Geometry check sheet. Reference: the model listing, model coordinates, mm. Face numbers are marked on the shaded views. Coordinates: 2 decimals unless noted, no trailing zeros. Order: outer loops, then holes, each group sorted by start corner. A loop starts at its lowest first (then second) coordinate and runs counter-clockwise, first axis right, second up. Notation, with made-up numbers: (-3, 80.25) - (4, 80.25) arc R22 ccw to (4, 117.25) - close; hole circle Ø11 at (-9, -39.5). An arc over 180 degrees is marked (long way). Put each result on its own line as item: value.
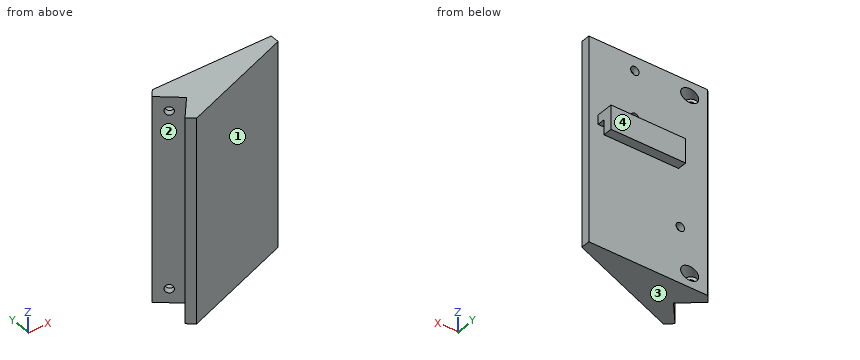
from build123d import *

# Parameters (mm, degrees)
EXTRUDE_1_DEPTH     = 65
EXTRUDE_2_DEPTH     = 5
EXTRUDE_4_DEPTH     = 8
SKETCH_9_R          = 2.3
CUT_EXTRUDE_4_DEPTH = 3.5
CUT_EXTRUDE_6_DEPTH = 14
EXTRUDE_5_DEPTH     = 40
HOLE_WIZARD_M4_1_D  = 4.5
CUT_EXTRUDE_START   = -3.5
SKETCH_17_R         = 3.75
CUT_EXTRUDE_7_DEPTH = 51.05954578
F_4_0MM_1_D         = 4.6
F_4_0MM_1_DEPTH     = 3.5
CUT_EXTRUDE_8_DEPTH = 5


with BuildPart() as part:
    # ｽｹｯﾁ1 → ﾎﾞｽ - 押し出し1 (new body)
    with BuildSketch(Plane.XY):
        Polygon((0, 0), (9.641814145, 11.490666647), (-1.848852501, 21.132480792), (1.365085547, 24.962703008), (65.946194887, 24.962703008), (65.946194887, 19.962703008), (3.830222216, -3.213938048), align=None)
    extrude(amount=EXTRUDE_1_DEPTH)

    # ｽｹｯﾁ6 → ﾎﾞｽ - 押し出し2 (add)
    with BuildSketch(Plane.XY.offset(65)):
        Polygon((0, 0), (3.830222216, -3.213938048), (65.946194887, 19.962703008), (65.946194887, 34.162703008), (9.084802154, 34.162703008), (-1.848852501, 21.132480792), (9.641814145, 11.490666647), align=None)
    extrude(amount=EXTRUDE_2_DEPTH)

    # ｽｹｯﾁ8 → ﾎﾞｽ - 押し出し4 (add)
    with BuildSketch(Plane(origin=(0, 0, 65), x_dir=(-1, 0, 0), z_dir=(0, 0, -1))):
        Polygon((-65.946194887, 34.162703008), (-65.946194887, 29.162703008), (-4.889303998, 29.162703008), (-9.084802154, 34.162703008), align=None)
    extrude(amount=EXTRUDE_4_DEPTH)

    # ｽｹｯﾁ9 → ｶｯﾄ - 押し出し4 (cut)
    with BuildSketch(Plane(origin=(0, 24.962703008, 0), x_dir=(1, 0, 0), z_dir=(0, 1, 0))):
        with Locations((16.255085547, -30)):
            Circle(SKETCH_9_R)
    extrude(amount=-CUT_EXTRUDE_4_DEPTH, mode=Mode.SUBTRACT)

    # ｽｹｯﾁ11 → ｶｯﾄ - 押し出し6 (cut, through all)
    with BuildSketch(Plane(origin=(0, 0, 57), x_dir=(-1, 0, 0), z_dir=(0, 0, -1))):
        Polygon((-1.365085547, 24.962703008), (-9.084802154, 34.162703008), (-20.364802154, 34.162703008), (-20.364802154, 24.962703008), align=None)
    extrude(amount=-CUT_EXTRUDE_6_DEPTH, mode=Mode.SUBTRACT)

    # ｽｹｯﾁ12 → ﾎﾞｽ - 押し出し5 (add)
    with BuildSketch(Plane.XY.offset(70)):
        Polygon((0, 0), (3.830222216, -3.213938048), (65.946194887, 19.962703008), (65.946194887, 24.962703008), (1.365085547, 24.962703008), (-1.848852501, 21.132480792), (9.641814145, 11.490666647), align=None)
    extrude(amount=EXTRUDE_5_DEPTH)

    # M4 すきま穴1 (through all)
    with Locations(Plane(origin=(9.641814145, 11.490666647, 0), x_dir=(-0.766044443, 0.64278761, 0), z_dir=(-0.64278761, -0.766044443, 0))):
        with Locations((7.5, -102.5), (7.5, -7.5)):
            Hole(HOLE_WIZARD_M4_1_D / 2)

    # ｽｹｯﾁ17 → ｶｯﾄ - 押し出し7 (cut, through all)
    with BuildSketch(Plane(origin=(9.641814145, 11.490666647, 0), x_dir=(0.766044443, -0.64278761, 0), z_dir=(-0.64278761, -0.766044443, 0)).offset(CUT_EXTRUDE_START)):
        with Locations((-7.5, 102.5)):
            Circle(SKETCH_17_R)
        with Locations((-7.5, 7.5)):
            Circle(SKETCH_17_R)
    extrude(amount=-CUT_EXTRUDE_7_DEPTH, mode=Mode.SUBTRACT)

    # Ø4.0mm ﾀﾞｳｴﾙ穴1
    with Locations(Plane(origin=(0, 24.962703008, 0), x_dir=(1, 0, 0), z_dir=(0, 1, 0))):
        with Locations((40.946194887, -77.5), (40.946194887, -102.5)):
            Hole(F_4_0MM_1_D / 2, depth=F_4_0MM_1_DEPTH)

    # ｽｹｯﾁ20 → ｶｯﾄ - 押し出し8 (cut)
    with BuildSketch(Plane(origin=(65.946194887, 0, 0), x_dir=(0, 0, -1), z_dir=(1, 0, 0))):
        Polygon((-70, 24.962703008), (-65, 24.962703008), (-65, 29.162703008), (-57, 29.162703008), (-57, 34.162703008), (-70, 34.162703008), align=None)
    extrude(amount=-CUT_EXTRUDE_8_DEPTH, mode=Mode.SUBTRACT)


solid = part.part
Q1. Section check C-C on x = 25. Record the boundary of the cut face in (y, z), then the cut area to 3 significant figures.
Answer block:
outline: (4.68, 0) - (24.96, 0) - (24.96, 65) - (29.16, 65) - (29.16, 57) - (34.16, 57) - (34.16, 70) - (24.96, 70) - (24.96, 110) - (4.68, 110) - close
area: 2,320 mm^2
Q2. Section check B-B on z = 102.5. Record the boundary of the cut face in (x, y), then the cut area to 3 significant figures.
Answer block:
outline: (-1.85, 21.13) - (2.17, 17.76) - (4.42, 20.44) - (3.27, 21.4) - (6.26, 24.96) - (1.37, 24.96) - close; (0, 0) - (3.83, -3.21) - (65.95, 19.96) - (65.95, 24.96) - (43.25, 24.96) - (43.25, 21.46) - (38.65, 21.46) - (38.65, 24.96) - (16.05, 24.96) - (9.02, 16.58) - (7.87, 17.55) - (5.62, 14.87) - (9.64, 11.49) - close
area: 950 mm^2
Q3. Draft check along Y on the marked faces 1, 2, 3 and 4. Enter one of: pulls with the +Y half, pulls with the -Y half, needs draft (parallel to the pull), parting line crosses it, or undercut.
Answer block:
face 1: pulls with the -Y half
face 2: undercut
face 3: needs draft
face 4: pulls with the +Y half
Q4. Section check A-A on z = 67.5. Record the boundary of the cut face in (x, y).
Answer block:
outline: (-1.85, 21.13) - (9.64, 11.49) - (0, 0) - (3.83, -3.21) - (65.95, 19.96) - (65.95, 24.96) - (60.95, 24.96) - (60.95, 34.16) - (20.36, 34.16) - (20.36, 24.96) - (1.37, 24.96) - close
Q5. Thickness scan on L1, parallel to Z at x = 5, y = 19; L2, parallel to Y at x = 57.5, z = 59; L3, parallel to Z at x = 32, y = 32.5. Record the ranges inside material, lowest first. Write a range as [from, to].
Answer block:
L1: z = [0, 5.43], [9.57, 100.43], [104.57, 110]
L2: y = [16.81, 24.96], [29.16, 34.16]
L3: z = [57, 70]
Q6. Section check D-D on z = 30. Record the boundary of the cut face in (x, y).
Answer block:
outline: (-1.85, 21.13) - (9.64, 11.49) - (0, 0) - (3.83, -3.21) - (65.95, 19.96) - (65.95, 24.96) - (18.56, 24.96) - (18.56, 21.46) - (13.96, 21.46) - (13.96, 24.96) - (1.37, 24.96) - close
Q7. Depth check by flat-ended pin: pin 1 Ø3 at (y, z) = (29.5, 63) entering from +X; pin 2 Ø3 at (x, z) = (13, 35) entering from -Y; pin 3 Ø1.3 at (x, y) = (33, 28) entering from -Z; pin 4 Ø12 at (x, y) = (47.5, 6) entering from +Z. Enter the tip coordinate at first touch or a pass-through.
Answer block:
pin 1: stops at x = 60.95
pin 2: stops at y = -0.35
pin 3: stops at z = 65
pin 4: passes through
